Can you work these out from the model? Positions are in its coordinate system, mm. A direction names the side the tool comes from. Round coordinates to 2 decimals unless told otherwise and drop trailing zeros. Loops run counter-clockwise (first coordinate to the right, second up) from the corner with the lowest first, then second, coordinate; pieces in that order, holes last.
```python
from build123d import *

# Parameters (mm, degrees)
SKETCH_1_W                   = 60
SKETCH_1_H                   = 88
EXTRUDE_1_DEPTH              = 6.8
SKETCH_2_R                   = 2.75
CUT_EXTRUDE_6_DEPTH          = 63.659715927
SKETCH_3_R                   = 11.05
CUT_EXTRUDE_7_DEPTH          = 3.2
SKETCH_4_R                   = 4.99
SKETCH_4_R_2                 = 2.75
EXTRUDE_2_DEPTH              = 8.2
SKETCH_5_R                   = 6
SKETCH_5_R_2                 = 4
EXTRUDE_1349_DEPTH           = 0.2
HOLE_WIZARD_M3_2_AT_2_COUNT  = 2
HOLE_WIZARD_M3_2_AT_2_PITCH  = 31
HOLE_WIZARD_M3_2_AT_3_COUNT  = 2
HOLE_WIZARD_M3_2_AT_3_PITCH  = 46.585942086
HOLE_WIZARD_M3_2_AT_4_COUNT  = 2
HOLE_WIZARD_M3_2_AT_4_PITCH  = 43.840620434
HOLE_WIZARD_M3_2_AT_5_COUNT  = 2
HOLE_WIZARD_M3_2_AT_5_PITCH  = 31
HOLE_WIZARD_M3_2_AT_6_COUNT  = 2
HOLE_WIZARD_M3_2_AT_6_PITCH  = 49.307707308
HOLE_WIZARD_M3_2_AT_7_COUNT  = 2
HOLE_WIZARD_M3_2_AT_7_PITCH  = 20.426698216
HOLE_WIZARD_M3_2_AT_8_COUNT  = 2
HOLE_WIZARD_M3_2_AT_8_PITCH  = 35.933967218
HOLE_WIZARD_M3_2_AT_9_COUNT  = 2
HOLE_WIZARD_M3_2_AT_9_PITCH  = 12.5
HOLE_WIZARD_M3_2_AT_10_COUNT = 2
HOLE_WIZARD_M3_2_AT_10_PITCH = 32.097507691
CUT_EXTRUDE_8_DEPTH          = 63.827064232
CUT_EXTRUDE_9_DEPTH          = 3.4
CHAMFER_1_SIZE               = 3.535533906


with BuildPart() as part:
    # 草图1 → 凸台-拉伸1 (new body)
    with BuildSketch(Plane(origin=(0, 0, 0), x_dir=(1, 0, 0), z_dir=(0, 1, 0))):
        with Locations((12, 2)):
            Rectangle(SKETCH_1_W, SKETCH_1_H)
    extrude(amount=EXTRUDE_1_DEPTH)

    # 草图2 → 切除-拉伸6 (cut, through all)
    with BuildSketch(Plane(origin=(0, 0, 0), x_dir=(1, 0, 0), z_dir=(0, 1, 0))):
        with Locations(Location((21, -21, 0), (0, 0, 270))):
            Circle(SKETCH_2_R)
        with BuildLine():
            Line((18.25, 21), (18.25, 25))
            ThreePointArc((18.25, 25), (21, 27.75), (23.75, 25))
            Line((23.75, 25), (23.75, 21))
            ThreePointArc((23.75, 21), (21, 18.25), (18.25, 21))
        make_face()
    extrude(amount=CUT_EXTRUDE_6_DEPTH, mode=Mode.SUBTRACT)

    # 草图3 → 切除-拉伸7 (cut)
    with BuildSketch(Plane.XZ):
        with Locations(Location((21, 21, 0), (0, 0, 270))):
            Circle(SKETCH_3_R)
        with BuildLine():
            Line((32.05, -21), (32.05, -25))
            ThreePointArc((32.05, -25), (21, -36.05), (9.95, -25))
            Line((9.95, -25), (9.95, -21))
            ThreePointArc((9.95, -21), (21, -9.95), (32.05, -21))
        make_face()
    extrude(amount=-CUT_EXTRUDE_7_DEPTH, mode=Mode.SUBTRACT)

    # 草图4 → 凸台-拉伸2 (add)
    with BuildSketch(Plane(origin=(0, 6.8, 0), x_dir=(1, 0, 0), z_dir=(0, 1, 0))):
        with Locations(Location((21, -21, 0), (0, 0, 270))):
            Circle(SKETCH_4_R)
        with Locations(Location((21, -21, 0), (0, 0, 90))):
            Circle(SKETCH_4_R_2, mode=Mode.SUBTRACT)
    extrude(amount=EXTRUDE_2_DEPTH)

    # 草图5 → Extrude 1349 (add)
    with BuildSketch(Plane(origin=(0, 6.8, 0), x_dir=(1, 0, 0), z_dir=(0, 1, 0))):
        with Locations(Location((21, -21, 0), (0, 0, 270))):
            Circle(SKETCH_5_R)
        with Locations((21, -21)):
            Circle(SKETCH_5_R_2, mode=Mode.SUBTRACT)
    extrude(amount=EXTRUDE_1349_DEPTH)

    # 草图8 → M3 六角凹头螺钉的柱形沉头孔2 (revolve, cut)
    with BuildSketch(Plane(origin=(5.5, 6.8, 5.5), x_dir=(0, 0, 1), z_dir=(1, 0, 0))):
        Polygon((0, 0), (0, 26.021463052), (1.7, 25), (1.7, 3.415021515), (1.725, 3.4), (3.25, 3.4), (3.25, 0), align=None)
    hole_wizard_m3_2 = revolve(axis=Axis((5.5, 13.15, 5.5), (0, -1, 0)), mode=Mode.SUBTRACT)

    # M3 六角凹头螺钉的柱形沉头孔2 at 2: M3 六角凹头螺钉的柱形沉头孔2 ×2
    with Locations(*[(i * HOLE_WIZARD_M3_2_AT_2_PITCH, 0, 0) for i in range(1, HOLE_WIZARD_M3_2_AT_2_COUNT)]):
        add(hole_wizard_m3_2, mode=Mode.SUBTRACT)

    # M3 六角凹头螺钉的柱形沉头孔2 at 3: M3 六角凹头螺钉的柱形沉头孔2 ×2
    with Locations(*[Vector(-0.21465703069033118, 0, -0.9766894896410068) * (i * HOLE_WIZARD_M3_2_AT_3_PITCH) for i in range(1, HOLE_WIZARD_M3_2_AT_3_COUNT)]):
        add(hole_wizard_m3_2, mode=Mode.SUBTRACT)

    # M3 六角凹头螺钉的柱形沉头孔2 at 4: M3 六角凹头螺钉的柱形沉头孔2 ×2
    with Locations(*[Vector(0.7071067811865475, 0, 0.7071067811865476) * (i * HOLE_WIZARD_M3_2_AT_4_PITCH) for i in range(1, HOLE_WIZARD_M3_2_AT_4_COUNT)]):
        add(hole_wizard_m3_2, mode=Mode.SUBTRACT)

    # M3 六角凹头螺钉的柱形沉头孔2 at 5: M3 六角凹头螺钉的柱形沉头孔2 ×2
    with Locations(*[(0, 0, i * HOLE_WIZARD_M3_2_AT_5_PITCH) for i in range(1, HOLE_WIZARD_M3_2_AT_5_COUNT)]):
        add(hole_wizard_m3_2, mode=Mode.SUBTRACT)

    # M3 六角凹头螺钉的柱形沉头孔2 at 6: M3 六角凹头螺钉的柱形沉头孔2 ×2
    with Locations(*[Vector(-0.38533529618817947, 0, -0.9227766303453767) * (i * HOLE_WIZARD_M3_2_AT_6_PITCH) for i in range(1, HOLE_WIZARD_M3_2_AT_6_COUNT)]):
        add(hole_wizard_m3_2, mode=Mode.SUBTRACT)

    # M3 六角凹头螺钉的柱形沉头孔2 at 7: M3 六角凹头螺钉的柱形沉头孔2 ×2
    with Locations(*[Vector(-0.9301552213313194, 0, -0.36716653473605715) * (i * HOLE_WIZARD_M3_2_AT_7_PITCH) for i in range(1, HOLE_WIZARD_M3_2_AT_7_COUNT)]):
        add(hole_wizard_m3_2, mode=Mode.SUBTRACT)

    # M3 六角凹头螺钉的柱形沉头孔2 at 8: M3 六角凹头螺钉的柱形沉头孔2 ×2
    with Locations(*[Vector(-0.5287476299210512, 0, 0.8487790901364567) * (i * HOLE_WIZARD_M3_2_AT_8_PITCH) for i in range(1, HOLE_WIZARD_M3_2_AT_8_COUNT)]):
        add(hole_wizard_m3_2, mode=Mode.SUBTRACT)

    # M3 六角凹头螺钉的柱形沉头孔2 at 9: M3 六角凹头螺钉的柱形沉头孔2 ×2
    with Locations(*[Vector(-0.7999999999999885, 0, -0.6000000000000153) * (i * HOLE_WIZARD_M3_2_AT_9_PITCH) for i in range(1, HOLE_WIZARD_M3_2_AT_9_COUNT)]):
        add(hole_wizard_m3_2, mode=Mode.SUBTRACT)

    # M3 六角凹头螺钉的柱形沉头孔2 at 10: M3 六角凹头螺钉的柱形沉头孔2 ×2
    with Locations(*[Vector(-0.3115506691716164, 0, 0.9502295409735051) * (i * HOLE_WIZARD_M3_2_AT_10_PITCH) for i in range(1, HOLE_WIZARD_M3_2_AT_10_COUNT)]):
        add(hole_wizard_m3_2, mode=Mode.SUBTRACT)

    # 草图9 → 切除-拉伸8 (cut, through all)
    with BuildSketch(Plane(origin=(0, 6.8, 0), x_dir=(1, 0, 0), z_dir=(0, 1, 0))):
        with BuildLine():
            Line((3.8, 5.5), (3.8, 9.5))
            ThreePointArc((3.8, 9.5), (5.5, 11.2), (7.2, 9.5))
            Line((7.2, 9.5), (7.2, 5.5))
            ThreePointArc((7.2, 5.5), (5.5, 3.8), (3.8, 5.5))
        make_face()
        with BuildLine():
            Line((34.8, 5.5), (34.8, 9.5))
            ThreePointArc((34.8, 9.5), (36.5, 11.2), (38.2, 9.5))
            Line((38.2, 9.5), (38.2, 5.5))
            ThreePointArc((38.2, 5.5), (36.5, 3.8), (34.8, 5.5))
        make_face()
        with BuildLine():
            Line((34.8, 36.5), (34.8, 40.5))
            ThreePointArc((34.8, 40.5), (36.5, 42.2), (38.2, 40.5))
            Line((38.2, 40.5), (38.2, 36.5))
            ThreePointArc((38.2, 36.5), (36.5, 34.8), (34.8, 36.5))
        make_face()
        with BuildLine():
            Line((3.8, 36.5), (3.8, 40.5))
            ThreePointArc((3.8, 40.5), (5.5, 42.2), (7.2, 40.5))
            Line((7.2, 40.5), (7.2, 36.5))
            ThreePointArc((7.2, 36.5), (5.5, 34.8), (3.8, 36.5))
        make_face()
    extrude(amount=-CUT_EXTRUDE_8_DEPTH, mode=Mode.SUBTRACT)

    # 草图10 → 切除-拉伸9 (cut)
    # profile 1 of 4: a face of its own
    with BuildSketch(Plane(origin=(0, 6.8, 0), x_dir=(1, 0, 0), z_dir=(0, 1, 0))):
        with BuildLine():
            Line((2.5, 5.5), (2.5, 9.5))
            ThreePointArc((2.5, 9.5), (5.5, 12.5), (8.5, 9.5))
            Line((8.5, 9.5), (8.5, 5.5))
            ThreePointArc((8.5, 5.5), (5.5, 2.5), (2.5, 5.5))
        make_face()
        with BuildLine():
            Line((7.2, 5.5), (7.2, 9.5))
            ThreePointArc((7.2, 9.5), (5.5, 11.2), (3.8, 9.5))
            Line((3.8, 9.5), (3.8, 5.5))
            ThreePointArc((3.8, 5.5), (5.5, 3.8), (7.2, 5.5))
        make_face(mode=Mode.SUBTRACT)
    # profile 2 of 4: a face of its own
    with BuildSketch(Plane(origin=(0, 6.8, 0), x_dir=(1, 0, 0), z_dir=(0, 1, 0))):
        with BuildLine():
            Line((33.5, 5.5), (33.5, 9.5))
            ThreePointArc((33.5, 9.5), (36.5, 12.5), (39.5, 9.5))
            Line((39.5, 9.5), (39.5, 5.5))
            ThreePointArc((39.5, 5.5), (36.5, 2.5), (33.5, 5.5))
        make_face()
        with BuildLine():
            Line((34.8, 9.5), (34.8, 5.5))
            ThreePointArc((34.8, 5.5), (36.5, 3.8), (38.2, 5.5))
            Line((38.2, 5.5), (38.2, 9.5))
            ThreePointArc((38.2, 9.5), (36.5, 11.2), (34.8, 9.5))
        make_face(mode=Mode.SUBTRACT)
    # profile 3 of 4: a face of its own
    with BuildSketch(Plane(origin=(0, 6.8, 0), x_dir=(1, 0, 0), z_dir=(0, 1, 0))):
        with BuildLine():
            Line((33.5, 36.5), (33.5, 40.5))
            ThreePointArc((33.5, 40.5), (36.5, 43.5), (39.5, 40.5))
            Line((39.5, 40.5), (39.5, 36.5))
            ThreePointArc((39.5, 36.5), (36.5, 33.5), (33.5, 36.5))
        make_face()
        with BuildLine():
            Line((38.2, 36.5), (38.2, 40.5))
            ThreePointArc((38.2, 40.5), (36.5, 42.2), (34.8, 40.5))
            Line((34.8, 40.5), (34.8, 36.5))
            ThreePointArc((34.8, 36.5), (36.5, 34.8), (38.2, 36.5))
        make_face(mode=Mode.SUBTRACT)
    # profile 4 of 4: a face of its own
    with BuildSketch(Plane(origin=(0, 6.8, 0), x_dir=(1, 0, 0), z_dir=(0, 1, 0))):
        with BuildLine():
            Line((2.5, 36.5), (2.5, 40.5))
            ThreePointArc((2.5, 40.5), (5.5, 43.5), (8.5, 40.5))
            Line((8.5, 40.5), (8.5, 36.5))
            ThreePointArc((8.5, 36.5), (5.5, 33.5), (2.5, 36.5))
        make_face()
        with BuildLine():
            Line((3.8, 40.5), (3.8, 36.5))
            ThreePointArc((3.8, 36.5), (5.5, 34.8), (7.2, 36.5))
            Line((7.2, 36.5), (7.2, 40.5))
            ThreePointArc((7.2, 40.5), (5.5, 42.2), (3.8, 40.5))
        make_face(mode=Mode.SUBTRACT)
    extrude(amount=-CUT_EXTRUDE_9_DEPTH, mode=Mode.SUBTRACT)

    # 倒角1
    chamfer_1_edges = [part.edges().sort_by_distance(p)[0] for p in [
        (-18, 3.4, -46),
        (42, 3.4, -46),
        (42, 3.4, 42),
        (-18, 3.4, 42),
    ]]
    chamfer(chamfer_1_edges, length=CHAMFER_1_SIZE)


solid = part.part
```
(1) Suppose I cut it at B-B (z = 21). Write out the boundary of the cut face in (x, y).
(2) Which directions (+Z, -Z, +X, -X, +Y, -Y) give clear straight access to the entire face, cutting with the end or side of a thin tool? Please do faces 4 (the flat face through (3.8, 2, -38)), 5 (the flat face through (33.5, 5, -7)), 6 (the flat face through (18.7, 3.2, 18.7)).
(3) Suppose I cut it at A-A (x = -13.5). Give the number of separate pieces and of enclosed holes in the cut face, then the cut area to 3 significant figures.
(4) If I drill on line 1 (X direction, y = 5.1, z = 5.5); line 2 (Z direction, x = 5.5, y = 1.7); line 3 (X direction, y = 5.55, z = -40), over which ranges is the centre line in solid material (lowest first)?
(5) For pin 1 (2.5 mm diameter, centred on x = -13.5, z = -40, fed in from -Y) (3 decimals); pin 2 (8.5 mm diameter, centred on x = -4.5, z = -2, fed in from +Y); pin 3 (4 mm diameter, centred on x = 5.5, z = 5.5, fed in from +Y), each with a flat end and sliding along its axis, tell me the tip position at first contact or that it passes through.
(6) Suppose I cut it at C-C (y = 9.5). Write out the boundary of the cut face in (x, z).
(7) We'd pull the mould along Z, two halves only. Please class faces 1 (the flat face through (42, 3, -1)), 2 (the flat face through (32.05, 2, -23)), 3 (the flat face through (40.257, 3.352, 40.207)): released by +Z, released by -Z, zero draft, split by the parting line, or undercut.
Check result:
1. outline: (-18, 0) - (9.95, 0) - (9.95, 3.2) - (18.25, 3.2) - (18.25, 15) - (16.01, 15) - (16.01, 7) - (15, 7) - (15, 6.8) - (-18, 6.8) - close; (23.75, 3.2) - (32.05, 3.2) - (32.05, 0) - (42, 0) - (42, 6.8) - (27, 6.8) - (27, 7) - (25.99, 7) - (25.99, 15) - (23.75, 15) - close
2. face 4: +Y, -Y
2. face 5: +Y
2. face 6: -Y
3. separate pieces: 4
3. enclosed holes: 0
3. area: 497 mm2
4. line 1: x = -18 to 2.25, 8.75 to 33.25, 39.75 to 42
4. line 2: z = -46 to -42.2, -34.8 to -11.2, -3.8 to 3.8, 7.2 to 34.8, 38.2 to 42
4. line 3: x = -18 to -16.75, -10.25 to -7.75, -1.25 to 2.5, 8.5 to 33.5, 39.5 to 42
5. pin 1: passes through
5. pin 2: stops at y = 6.8
5. pin 3: stops at y = 3.4
6. outline: circle Ø9.98 at (21, 21); hole circle Ø5.5 at (21, 21)
7. face 1: zero draft
7. face 2: undercut
7. face 3: released by +Z
